Could you check a few things on this model? Use its own coordinates, in mm. Face numbers are marked on the shaded views. Give positions to 0.01 mm unless a question says otherwise; leave off trailing zeros. Write each loop counter-clockwise with the first axis right and the second up, starting at its lowest first coordinate (ties: lowest second). Pieces come first, ordered by that corner, then holes. Notation, with made-up numbers: (-22, -35.75) - (20, -35.75) arc R11 cw to (20, -28.75) - close; hole circle Ø11 at (-13.5, 10.25). An arc over 180 degrees is marked (long way). Answer in a Markdown table with one row per item.
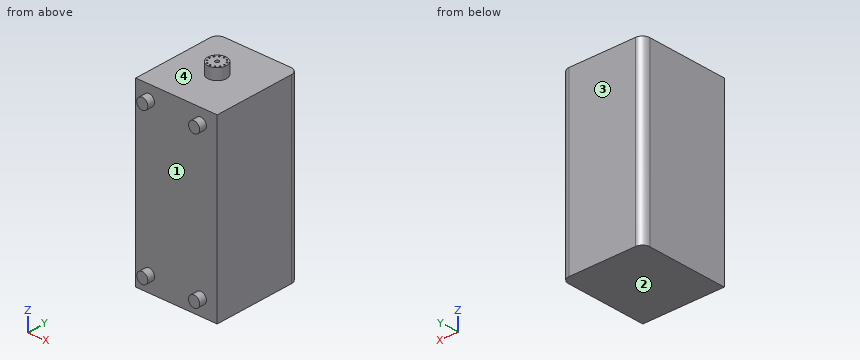
from build123d import *

# Parameters (mm, degrees)
SKETCH1_W           = 110
SKETCH1_H           = 120
BOSS_EXTRUDE1_DEPTH = 240
FILLET1_R           = 10
SKETCH2_R           = 7.5
BOSS_EXTRUDE2_DEPTH = 10
SKETCH3_R           = 12.7
SKETCH3_R_2         = 2.516719654
SKETCH3_R_3         = 1
BOSS_EXTRUDE3_DEPTH = 15


with BuildPart() as part:
    # Sketch1 → Boss-Extrude1 (new body)
    with BuildSketch(Plane.XY):
        Rectangle(SKETCH1_W, SKETCH1_H)
    extrude(amount=BOSS_EXTRUDE1_DEPTH)

    # Fillet1
    fillet1_edges = [part.edges().sort_by_distance(p)[0] for p in [
        (-55, 60, 120),
        (55, 60, 120),
    ]]
    fillet(fillet1_edges, radius=FILLET1_R)

    # Sketch2 → Boss-Extrude2 (add)
    with BuildSketch(Plane.XZ.offset(60)):
        with Locations(Location((-37.059126993, 221.569070344, 0), (0, 0, 180))):
            Circle(SKETCH2_R)
        with Locations(Location((32.940873007, 221.569070344, 0), (0, 0, 180))):
            Circle(SKETCH2_R)
        with Locations(Location((32.940873007, 21.569070344, 0), (0, 0, 180))):
            Circle(SKETCH2_R)
        with Locations(Location((-37.059126993, 21.569070344, 0), (0, 0, 180))):
            Circle(SKETCH2_R)
    extrude(amount=BOSS_EXTRUDE2_DEPTH)

    # Sketch3 → Boss-Extrude3 (add)
    with BuildSketch(Plane.XY.offset(240)):
        Circle(SKETCH3_R)
        Circle(SKETCH3_R_2, mode=Mode.SUBTRACT)
        with Locations((-10.265012075, 0)):
            Circle(SKETCH3_R_3, mode=Mode.SUBTRACT)
        with Locations((-8.889761227, 5.132506037)):
            Circle(SKETCH3_R_3, mode=Mode.SUBTRACT)
        with Locations((-5.132506037, 8.889761227)):
            Circle(SKETCH3_R_3, mode=Mode.SUBTRACT)
        with Locations((0, 10.265012075)):
            Circle(SKETCH3_R_3, mode=Mode.SUBTRACT)
        with Locations((5.132506037, 8.889761227)):
            Circle(SKETCH3_R_3, mode=Mode.SUBTRACT)
        with Locations((8.889761227, 5.132506037)):
            Circle(SKETCH3_R_3, mode=Mode.SUBTRACT)
        with Locations((10.265012075, 0)):
            Circle(SKETCH3_R_3, mode=Mode.SUBTRACT)
        with Locations((8.889761227, -5.132506037)):
            Circle(SKETCH3_R_3, mode=Mode.SUBTRACT)
        with Locations((5.132506037, -8.889761227)):
            Circle(SKETCH3_R_3, mode=Mode.SUBTRACT)
        with Locations((0, -10.265012075)):
            Circle(SKETCH3_R_3, mode=Mode.SUBTRACT)
        with Locations((-5.132506037, -8.889761227)):
            Circle(SKETCH3_R_3, mode=Mode.SUBTRACT)
        with Locations((-8.889761227, -5.132506037)):
            Circle(SKETCH3_R_3, mode=Mode.SUBTRACT)
    extrude(amount=BOSS_EXTRUDE3_DEPTH)


solid = part.part
1) Imagine slicing it at B-B (y = -41.5). List the corners of the cut face in (x, z) for me, then the cut area to 3 significant figures.
Check values:
| item | result |
|---|---|
| outline | (-55, 0) - (55, 0) - (55, 240) - (-55, 240) - close |
| area | 26,400 mm2 |
2) Will these pins go through, and if not, where does the flat tip stop? P1, Ø8, axis at x = -20.5, y = -50.5, coming from the +Z side; P2, Ø3, axis at x = 0, y = -10.27, coming from the +Z side; P3, Ø12, axis at x = -3, z = 140.5, coming from the -Y side.
Check values:
| item | result |
|---|---|
| P1 | stops at z = 240 |
| P2 | stops at z = 255 |
| P3 | stops at y = -60 |
3) If I drill on line 1 (Y direction, x = 0, z = 249); line 2 (Z direction, x = 40, y = 38); line 3 (Y direction, x = -10, z = 104), over which ranges is the centre line in solid material (lowest first)?
Check values:
| item | result |
|---|---|
| line 1 | y = -12.7 to -11.27, -9.27 to -2.52, 2.52 to 9.27, 11.27 to 12.7 |
| line 2 | z = 0 to 240 |
| line 3 | y = -60 to 60 |
4) Imagine slicing it at C-C (x = 47.5). List the corners of the cut face in (y, z) for me.
Check values:
| item | result |
|---|---|
| outline | (-60, 0) - (59.68, 0) - (59.68, 240) - (-60, 240) - close |
5) We'd pull the mould along Z, two halves only. Please class the marked faces 1, 2, 3 and 4: +Z half, -Z half, draft (parallel to the pull), parting line (faces both ways), or undercut.
Check values:
| item | result |
|---|---|
| face 1 | undercut |
| face 2 | -Z half |
| face 3 | draft |
| face 4 | +Z half |
6) Imagine slicing it at A-A (z = 52). List the corners of the cut face in (x, y) for me, then the cut area to 3 significant figures.
Check values:
| item | result |
|---|---|
| outline | (-55, -60) - (55, -60) - (55, 50) arc R10 ccw to (45, 60) - (-45, 60) arc R10 ccw to (-55, 50) - close |
| area | 13,200 mm2 |
